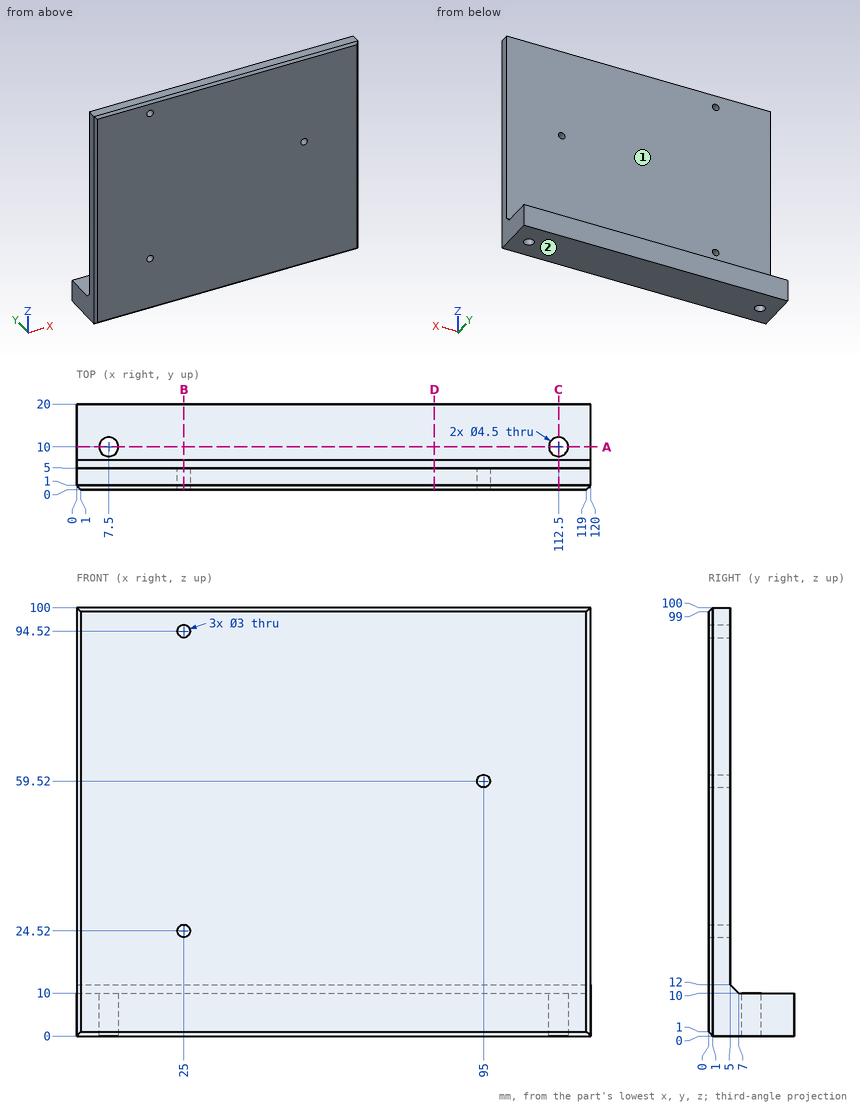
Here's the drawing with two shaded views (mm, measured from the low corner). I have some questions. A direction names the side the tool comes from. Give positions to 0.01 mm unless a question says otherwise; leave off trailing zeros. Write each loop counter-clockwise with the first axis right and the second up, starting at its lowest first coordinate (ties: lowest second). Pieces come first, ordered by that corner, then holes. Notation, with made-up numbers: (-17.5, -18.75) - (39.5, -18.75) arc R20 ccw to (39.5, -12.75) - close; hole circle Ø11 at (-23.75, 89). An arc over 180 degrees is marked (long way). One line per item, written item: value. Start each with the question number.
Item 1: Imagine slicing it at D-D, the plane x = 83.5. List the corners of the cut face in (y, z) for me.
Item 2: I'm going to push flat-ended pins straight in: pin 1 (5 mm diameter, centred on x = 95, z = 59.52, fed in from +Y); pin 2 (10.5 mm diameter, centred on x = 50, y = 13, fed in from +Z). Where does each tip first touch, or does it pass through?
Item 3: Imagine slicing it at B-B, the plane x = 25. List the corners of the cut face in (y, z) for me, and give its area (3 significant figures).
Item 4: Imagine slicing it at A-A, the plane y = 10. List the corners of the cut face in (x, z) for me, and give its area (3 significant figures).
Item 5: Which directions (+Z, -Z, +X, -X, +Y, -Y) give clear straight access to the entire face, cutting with the end or side of a thin tool? Please do the marked faces 1 and 2.
Item 6: Imagine slicing it at C-C, the plane x = 112.5. List the corners of the cut face in (y, z) for me.
Item 7: Please list where these lines run through material, in increasing order: line 1 (Z direction, x = 25, y = 3.8); line 2 (Y direction, x = 16.5, z = 95.5); line 3 (Z direction, x = 107, y = 8.5). Write a range as from..to.
Geometry says:
1. outline: (0, 1) - (1, 0) - (20, 0) - (20, 10) - (7, 10) - (5, 12) - (5, 100) - (1, 100) - (0, 99) - close
2. pin 1: y = 5
2. pin 2: z = 10
3. outline: (0, 1) - (1, 0) - (20, 0) - (20, 10) - (7, 10) - (5, 12) - (5, 23.02) - (0, 23.02) - close; (0, 26.02) - (5, 26.02) - (5, 93.02) - (0, 93.02) - close; (0, 96.02) - (5, 96.02) - (5, 100) - (1, 100) - (0, 99) - close
3. area: 621 mm^2
4. outline: (0, 0) - (5.25, 0) - (5.25, 10) - (0, 10) - close; (9.75, 0) - (110.25, 0) - (110.25, 10) - (9.75, 10) - close; (114.75, 0) - (120, 0) - (120, 10) - (114.75, 10) - close
4. area: 1,110 mm^2
5. face 1: +Z, +X, -X, +Y
5. face 2: -Z, +X, -X, +Y, -Y
6. outline: (0, 1) - (1, 0) - (7.75, 0) - (7.75, 10) - (7, 10) - (5, 12) - (5, 100) - (1, 100) - (0, 99) - close; (12.25, 0) - (20, 0) - (20, 10) - (12.25, 10) - close
7. line 1: 0..23.02, 26.02..93.02, 96.02..100
7. line 2: 0..5
7. line 3: 0..10
